from build123d import *

# Parameters (mm, degrees)
SKETCH1_W             = 46
SKETCH1_H             = 50
BOSS_EXTRUDE1_DEPTH   = 3
SKETCH2_W             = 3
SKETCH2_H             = 15
CUT_EXTRUDE1_DEPTH    = 53.999062732
LPATTERN1_COUNT       = 3
LPATTERN1_PITCH       = 22.8
SKETCH3_W             = 7.8
SKETCH3_H             = 3
BOSS_EXTRUDE2_DEPTH   = 3
LPATTERN2_COUNT       = 2
LPATTERN2_PITCH       = 22.8
F_6_CLEARANCE_HOLE1_D = 3.7973


with BuildPart() as part:
    # Sketch1 → Boss-Extrude1 (new body)
    with BuildSketch(Plane.XY):
        with Locations((-17.993460648, -8.457986111)):
            Rectangle(SKETCH1_W, SKETCH1_H)
    extrude(amount=BOSS_EXTRUDE1_DEPTH)

    # Sketch2 → Cut-Extrude1 (cut, through all)
    with BuildSketch(Plane.XY.offset(3)):
        with Locations((-39.493460648, 1.242013889)):
            Rectangle(SKETCH2_W, SKETCH2_H)
        with Locations((3.506539352, 1.242013889)):
            Rectangle(SKETCH2_W, SKETCH2_H)
    cut_extrude1 = extrude(amount=-CUT_EXTRUDE1_DEPTH, mode=Mode.SUBTRACT)

    # LPattern1: Cut-Extrude1 ×3
    with Locations(*[(0, -i * LPATTERN1_PITCH, 0) for i in range(1, LPATTERN1_COUNT)]):
        add(cut_extrude1, mode=Mode.SUBTRACT)

    # Sketch3 → Boss-Extrude2 (add)
    with BuildSketch(Plane(origin=(0, 16.542013889, 0), x_dir=(1, 0, 0), z_dir=(0, 1, 0))):
        with Locations((-29.393460648, -1.5)):
            Rectangle(SKETCH3_W, SKETCH3_H)
    boss_extrude2 = extrude(amount=BOSS_EXTRUDE2_DEPTH)

    # LPattern2: Boss-Extrude2 ×2
    with Locations(*[(i * LPATTERN2_PITCH, 0, 0) for i in range(1, LPATTERN2_COUNT)]):
        add(boss_extrude2)

    # #6 Clearance Hole1 (through all)
    with Locations(Plane.XY.offset(3)):
        with Locations((-8.993460648, -20.657986111), (-26.993460648, -20.657986111)):
            Hole(F_6_CLEARANCE_HOLE1_D / 2)


solid = part.part
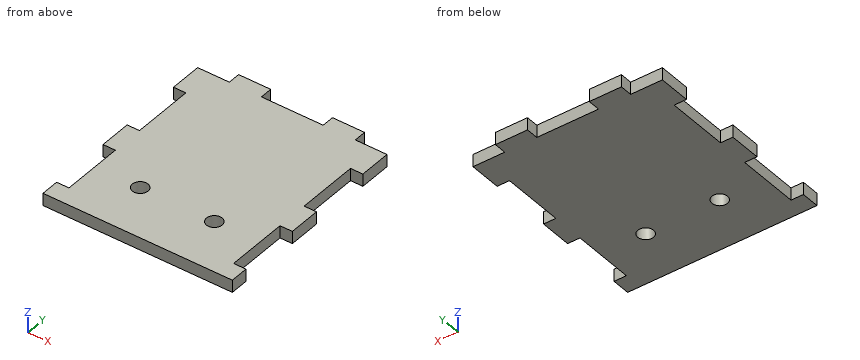
The listing builds one solid part. Answer for the finished solid, in the listing's coordinates (mm). Round coordinates to 2 decimals unless told otherwise and drop trailing zeros. Write each loop counter-clockwise with the first axis right and the second up, starting at its lowest first coordinate (ties: lowest second). Pieces come first, ordered by that corner, then holes. Notation, with made-up numbers: M 83.25,-39.5 L 115.25,-39.5 A28 ccw 115.25,-19.5 Z; hole C -39,75.5 d5. An arc over 180 degrees is marked long. Write each question's results on one line, items separated by ' | '. Start each with the question number.
Item 1: A cutting plane is placed at D-D on x = -35.5. Write down the section's boundary in (y, z).
Item 2: A cutting plane is placed at C-C on y = -25. Write down the section's boundary in (x, z).
Item 3: Straight lines are drawn through the part: L1, parallel to Y at x = -9, z = 0.75; L2, parallel to X at y = -21.5, z = 2.05; L3, parallel to X at y = -19, z = 2.45. For each, find the intervals that lie inside material, in ascending order. Write a range as [from, to].
Item 4: A cutting plane is placed at B-B on x = -28. Write down the section's boundary in (y, z), and give its area (3 significant figures).
Item 5: A cutting plane is placed at A-A on z = 0.75. State how many separate pieces and enclosed holes the cut face has, and give its area (3 significant figures).
Item 6: Flat-ended cylindrical pins translate along their axes: pin 1 Ø1.5 at (y, z) = (17.5, 1.5) entering from -X; pin 2 Ø0.9 at (x, z) = (4, 2) entering from +Y; pin 3 Ø0.9 at (y, z) = (-1.5, 2) entering from -X. Find the tip coordinate at first contact, or state that the pin passes through.
Check sheet entries:
1) outline: M -33.46,0 L 16.54,0 L 16.54,3 L -33.46,3 Z
2) outline: M -37.99,0 L 2.01,0 L 2.01,3 L -37.99,3 Z
3) L1: [-33.46, -22.56], [-18.76, 19.54] | L2: [-37.99, -28.7], [-25.29, -10.7], [-7.29, 2.01] | L3: [-37.99, -27.92], [-26.07, -9.92], [-8.07, 2.01]
4) outline: M -33.46,0 L -22.27,0 L -22.27,3 L -33.46,3 Z; M -19.05,0 L 19.54,0 L 19.54,3 L -19.05,3 Z | area: 149 mm²
5) separate pieces: 1 | enclosed holes: 2 | area: 2,140 mm²
6) pin 1: x = -33.29 | pin 2: y = 16.54 | pin 3: x = -37.99
